Study the drawing (mm; zero at the part's minimum x, y, z) and answer. Coordinates: 2 decimals unless noted, no trailing zeros. Loops run counter-clockwise (first coordinate to the right, second up) from the corner with the lowest first, then second, coordinate; pieces in that order, holes last. Notation, with made-up numbers: M 21.25,-30 L 45.25,-30 A16 ccw 45.25,-1 Z; hole C -24.75,50.25 d2. An arc over 180 degrees is marked long. Use one line per item in the form item = value. Start each with the question number.
1. The part is cut by section C-C (x = 100). Give the vertices of the cut face in (y, z) (1 decimal).
2. Flat-ended cylindrical pins translate along their axes: pin 1 (1 mm diameter, centred on x = 21.5, z = 60, fed in from -Y); pin 2 (2.5 mm diameter, centred on x = 104, z = 24.5, fed in from +Y). Find the tip coordinate at first contact, or state that the pin passes through.
3. The part is cut by section D-D (z = 36.5). Give the vertices of the cut face in (x, y) (1 decimal), plus the area to 3 significant figures.
4. The part is cut by section A-A (z = 10). Give the vertices of the cut face in (x, y) (3 decimals).
5. Find the intervals of material crossed by probe 1 along Z at (x, y) = (190, 2.45) (3 decimals); probe 2 along Z at (x, y) = (10, 3.1) (3 decimals); probe 3 along X at (y, z) = (2.15, 63) (3 decimals), in increasing order. Write a range as [from, to].
6. The part is cut by section B-B (y = 3.8). Give the number of separate pieces and of enclosed holes in the cut face, plus the area to 4 significant figures.
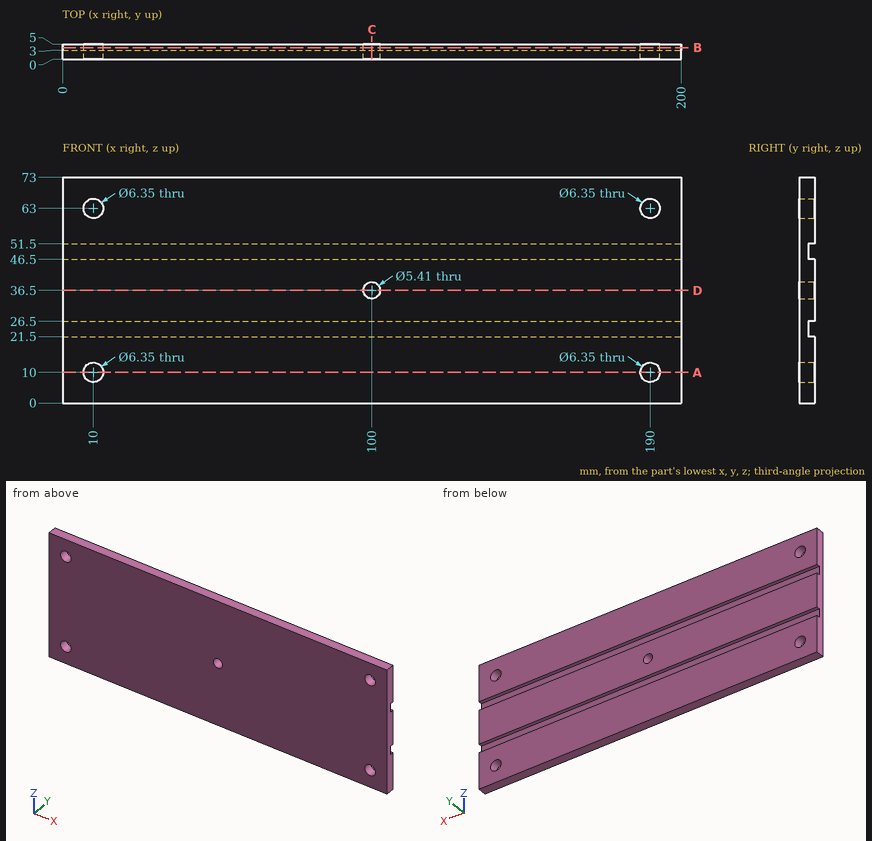
Computed values:
q1.outline = M 0,0 L 5,0 L 5,21.5 L 3,21.5 L 3,26.5 L 5,26.5 L 5,33.8 L 0,33.8 Z; M 0,39.2 L 5,39.2 L 5,46.5 L 3,46.5 L 3,51.5 L 5,51.5 L 5,73 L 0,73 Z
q2.pin_1 = 0
q2.pin_2 = 3
q3.outline = M 0,0 L 97.3,0 L 97.3,5 L 0,5 Z; M 102.7,0 L 200,0 L 200,5 L 102.7,5 Z
q3.area = 973 mm²
q4.outline = M 0,0 L 6.825,0 L 6.825,5 L 0,5 Z; M 13.175,0 L 186.825,0 L 186.825,5 L 13.175,5 Z; M 193.175,0 L 200,0 L 200,5 L 193.175,5 Z
q5.probe_1 = [0, 6.825], [13.175, 59.825], [66.175, 73]
q5.probe_2 = [0, 6.825], [13.175, 21.5], [26.5, 46.5], [51.5, 59.825], [66.175, 73]
q5.probe_3 = [0, 6.825], [13.175, 186.825], [193.175, 200]
q6.separate_pieces = 3
q6.enclosed_holes = 5
q6.area = 12,450 mm²
